from build123d import *

# Parameters (mm, degrees)
BOSS_EXTRUDE1_DEPTH = 10
SKETCH3_R           = 2.8067
CUT_EXTRUDE1_DEPTH  = 59.416607228
FILLET1_R           = 2.5
CIRPATTERN3_COUNT   = 3
CIRPATTERN3_ANGLE   = 180


with BuildPart() as part:
    # Sketch1 → Boss-Extrude1 (new body)
    with BuildSketch(Plane.XY):
        Polygon((-44.5, -6), (-38.5, -6), (-38.5, 13), (-21, 30.5), (21, 30.5), (38.5, 13), (38.5, -6), (44.5, -6), (44.5, 15.485281374), (23.485281374, 36.5), (-23.485281374, 36.5), (-44.5, 15.485281374), align=None)
    extrude(amount=BOSS_EXTRUDE1_DEPTH)

    # Sketch3 → Cut-Extrude1 (cut, through all)
    with BuildSketch(Plane(origin=(0, 0, 0), x_dir=(0, 0, -1), z_dir=(1, 0, 0))):
        with Locations(Location((-5, 0, 0), (0, 0, 90))):
            Circle(SKETCH3_R)
    cut_extrude1 = extrude(amount=CUT_EXTRUDE1_DEPTH, mode=Mode.SUBTRACT)

    # Fillet1
    fillet1_edges = [part.edges().sort_by_distance(p)[0] for p in [
        (38.5, -6, 5),
        (-38.5, -6, 5),
    ]]
    fillet(fillet1_edges, radius=FILLET1_R)

    # CirPattern3: Cut-Extrude1 ×3 about axis
    cirpattern3_axis = Axis((0, 0, 0), (0, 0, 1))
    for i in range(1, CIRPATTERN3_COUNT):
        add(cut_extrude1.rotate(cirpattern3_axis, i * CIRPATTERN3_ANGLE / (CIRPATTERN3_COUNT - 1)), mode=Mode.SUBTRACT)


solid = part.part
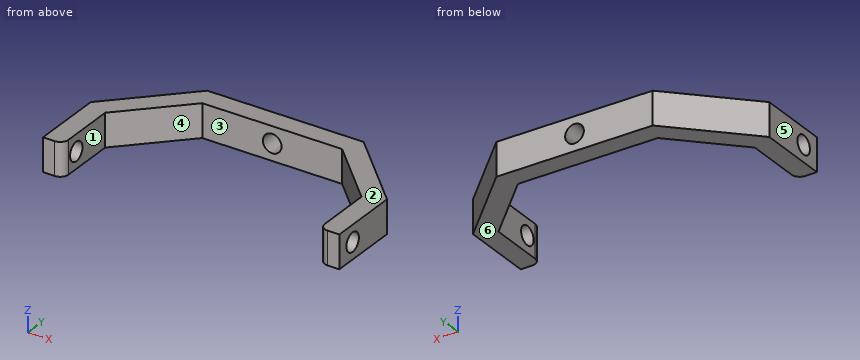
Geometry check sheet. Reference: the model listing, model coordinates, mm. Face numbers are marked on the shaded views. A direction names the side the tool comes from. Round coordinates to 2 decimals unless told otherwise and drop trailing zeros. Write each loop counter-clockwise with the first axis right and the second up, starting at its lowest first coordinate (ties: lowest second). Pieces come first, ordered by that corner, then holes. Notation, with made-up numbers: (-11.5, 64) -> (38.5, 64) arc R27 ccw to (38.5, 99) -> close; hole circle Ø10 at (54.5, 13). An arc over 180 degrees is marked (long way). One line per item, written item: value. Start each with the question number.
(1) Go/stop test with flat-tipped pins: pin 1 Ø4.5 at (y, z) = (0, 5) entering from -X; pin 2 Ø4 at (x, z) = (-23, 5.5) entering from -Y; pin 3 Ø4 at (x, z) = (-35, 6) entering from -Y; pin 4 Ø5 at (y, z) = (25.5, 6.5) entering from +X. Record where each tip stops, or that it passes through.
(2) Cross-section at C-C, the plane x = 0. Record the cut outline in (y, z), and give its area (3 significant figures).
(3) Scan lines: line 1 (X direction, y = 12.5, z = 1.25); line 2 (Z direction, x = -42.35, y = 0); line 3 (X direction, y = 22, z = 8.75). Record each from-to range of solid material in increasing order. Write a range as [from, to].
(4) Cross-section at B-B, the plane z = 5. Record the cut outline in (x, y).
(5) Cross-section at D-D, the plane y = 27. Record the cut outline in (x, z), and give its area (3 significant figures).
(6) Draft check along X on the marked faces 3, 4, 5 and 6. Enter one of: +X half, -X half, draft (parallel to the pull), parting line (faces both ways), or undercut.
(7) Cross-section at A-A, the plane y = 0. Record the cut outline in (x, z), and give its area (3 significant figures).
(8) Access from +Z, -Z, +X, -X, +Y, -Y to the whole of each face (thin tool, end or side, straight path). Record for the marked faces 1 and 2.
Answer:
1. pin 1: through
1. pin 2: y = 26.5
1. pin 3: y = 14.5
1. pin 4: x = 36.99
2. outline: (30.5, 0) -> (36.5, 0) -> (36.5, 2.19) -> (30.5, 2.19) -> close; (30.5, 7.81) -> (36.5, 7.81) -> (36.5, 10) -> (30.5, 10) -> close
2. area: 26.3 mm²
3. line 1: [-44.5, -38.5], [38.5, 44.5]
3. line 2: [0, 2.19], [7.81, 10]
3. line 3: [-37.99, -29.5], [29.5, 37.99]
4. outline: (-44.5, -6) -> (-41, -6) arc R2.5 ccw to (-38.5, -3.5) -> (-38.5, -2.81) -> (-44.5, -2.81) -> close; (-44.5, 2.81) -> (-38.5, 2.81) -> (-38.5, 13) -> (-21, 30.5) -> (-2.81, 30.5) -> (-2.81, 36.5) -> (-23.49, 36.5) -> (-44.5, 15.49) -> close; (2.81, 30.5) -> (21, 30.5) -> (38.5, 13) -> (38.5, 2.81) -> (44.5, 2.81) -> (44.5, 15.49) -> (23.49, 36.5) -> (2.81, 36.5) -> close; (38.5, -3.5) arc R2.5 ccw to (41, -6) -> (44.5, -6) -> (44.5, -2.81) -> (38.5, -2.81) -> close
5. outline: (-32.99, 0) -> (-24.5, 0) -> (-24.5, 10) -> (-32.99, 10) -> close; (24.5, 0) -> (32.99, 0) -> (32.99, 10) -> (24.5, 10) -> close
5. area: 170 mm²
6. face 3: undercut
6. face 4: undercut
6. face 5: -X half
6. face 6: draft
7. outline: (-44.5, 0) -> (-38.5, 0) -> (-38.5, 2.19) -> (-44.5, 2.19) -> close; (-44.5, 7.81) -> (-38.5, 7.81) -> (-38.5, 10) -> (-44.5, 10) -> close; (38.5, 0) -> (44.5, 0) -> (44.5, 2.19) -> (38.5, 2.19) -> close; (38.5, 7.81) -> (44.5, 7.81) -> (44.5, 10) -> (38.5, 10) -> close
7. area: 52.6 mm²
8. face 1: +Z, -Z, -Y
8. face 2: +Z, +X, -X, +Y, -Y
